```python
from build123d import *

# Parameters (mm, degrees)
SKETCH1_W           = 50
SKETCH1_H           = 10
BOSS_EXTRUDE1_DEPTH = 4
CUT_EXTRUDE1_DEPTH  = 2
CUT_EXTRUDE2_REACH  = 27.573
SKETCH3_R           = 1
CUT_EXTRUDE3_REACH  = 27.807
SKETCH4_W           = 8.712551382
SKETCH4_H           = 15.185608923
SKETCH5_W           = 19.235166375
SKETCH5_H           = 10
BOSS_EXTRUDE2_DEPTH = 4
FILLET1_R           = 10
FILLET2_R           = 2
FILLET3_R           = 2
FILLET4_R           = 2


with BuildPart() as part:
    # Sketch1 → Boss-Extrude1 (new body)
    with BuildSketch(Plane.XY):
        Rectangle(SKETCH1_W, SKETCH1_H)
    extrude(amount=BOSS_EXTRUDE1_DEPTH)

    # Sketch2 → Cut-Extrude1 (cut)
    with BuildSketch(Plane.XY.offset(4)):
        with BuildLine():
            Line((-2.254530133, 2.677142857), (-14.2, 2))
            ThreePointArc((-14.2, 2), (-16.2, 0), (-14.2, -2))
            Line((-14.2, -2), (-2.254530133, -2.677142857))
            ThreePointArc((-2.254530133, -2.677142857), (0, -3.5), (2.254530133, -2.677142857))
            Line((2.254530133, -2.677142857), (14.2, -2))
            ThreePointArc((14.2, -2), (16.2, 0), (14.2, 2))
            Line((14.2, 2), (2.254530133, 2.677142857))
            ThreePointArc((2.254530133, 2.677142857), (0, 3.5), (-2.254530133, 2.677142857))
        make_face()
    extrude(amount=-CUT_EXTRUDE1_DEPTH, mode=Mode.SUBTRACT)

    # Sketch3 → Cut-Extrude2 (cut, up to next)
    with BuildSketch(Plane.XY.offset(2), mode=Mode.PRIVATE) as cut_extrude2_sk1:
        with Locations((-14.45, 0)):
            Circle(SKETCH3_R)
    cut_extrude2_tool1 = extrude(cut_extrude2_sk1.sketch, amount=-CUT_EXTRUDE2_REACH, mode=Mode.PRIVATE) & part.part
    # Sketch3 → Cut-Extrude2 (cut, up to next)
    with BuildSketch(Plane.XY.offset(2), mode=Mode.PRIVATE) as cut_extrude2_sk2:
        with Locations(Location((14.45, 0, 0), (0, 0, 180))):
            Circle(SKETCH3_R)
    cut_extrude2_tool2 = extrude(cut_extrude2_sk2.sketch, amount=-CUT_EXTRUDE2_REACH, mode=Mode.PRIVATE) & part.part
    add(cut_extrude2_tool1.solids().sort_by_distance((-14.45, 0, 2))[0], mode=Mode.SUBTRACT)
    add(cut_extrude2_tool2.solids().sort_by_distance((14.45, 0, 2))[0], mode=Mode.SUBTRACT)

    # Sketch4 → Cut-Extrude3 (cut, up to next)
    with BuildSketch(Plane.XY.offset(4), mode=Mode.PRIVATE) as cut_extrude3_sk1:
        with Locations((-21.977833235, -0.132061848)):
            Rectangle(SKETCH4_W, SKETCH4_H)
    cut_extrude3_tool1 = extrude(cut_extrude3_sk1.sketch, amount=-CUT_EXTRUDE3_REACH, mode=Mode.PRIVATE) & part.part
    add(cut_extrude3_tool1.solids().sort_by_distance((-21.977833, -0.132062, 4))[0], mode=Mode.SUBTRACT)

    # Sketch5 → Boss-Extrude2 (add)
    with BuildSketch(Plane.XY.offset(4)):
        with Locations((34.617583188, 0)):
            Rectangle(SKETCH5_W, SKETCH5_H)
    extrude(amount=-BOSS_EXTRUDE2_DEPTH)

    # Fillet1
    fillet1_edges = [part.edges().sort_by_distance(p)[0] for p in [
        (44.235166375, 5, 2),
    ]]
    fillet(fillet1_edges, radius=FILLET1_R - 0.0001)  # a hair under: the kernel refuses the full size

    # Fillet2
    fillet2_edges = [part.edges().sort_by_distance(p)[0] for p in [
        (44.235166375, -5, 2),
    ]]
    fillet(fillet2_edges, radius=FILLET2_R)

    # Fillet3
    fillet3_edges = [part.edges().sort_by_distance(p)[0] for p in [
        (-17.621557544, 5, 2),
    ]]
    fillet(fillet3_edges, radius=FILLET3_R)

    # Fillet4
    fillet4_edges = [part.edges().sort_by_distance(p)[0] for p in [
        (-17.621557544, -5, 2),
    ]]
    fillet(fillet4_edges, radius=FILLET4_R)


solid = part.part
```
Read the model definition and answer for the solid it produces. Units are mm, in the model's axes. A direction names the side the tool comes from. Give positions to 0.01 mm unless a question says otherwise; leave off trailing zeros. Order: outer loops, then holes, each group sorted by start corner. A loop starts at its lowest first (then second) coordinate and runs counter-clockwise, first axis right, second up.
(1) Find section A-A (x = -11). Give the vertices of the cut face in (y, z), plus the area to 3 significant figures.
(2) Straight lines are drawn through the part: L1, parallel to Y at x = -14.45, z = 1.55; L2, parallel to X at y = -0.25, z = 1.9; L3, parallel to Z at x = 8, y = 2. For each, find the intervals that lie inside material, in ascending order.
(3) For faces 1 (the flat face through (0, 0, 2)), 2 (the cylindrical face through (-13.496, 0.3, 1.014)), determine the directions among +Z, -Z, +X, -X, +Y, -Y from which every point of the face is accessible in a straight line to the end or side of a thin tool.
(4) For a pull along Y with two mould halves and no side action, classify faces 3 (the flat face through (-17.622, 0, 2)), 4 (the cylindrical face through (-17.02, 4.43, 2.03)), 5 (the cylindrical face through (0, -3.5, 3)), 6 (the flat face through (-8.311, -2.334, 3.014)) as released by +Y, released by -Y, zero draft, split by the parting line, or undercut.
(5) Find section B-B (x = 4.5). Give the vertices of the cut face in (y, z).
(6) Given pin 1 (1.5 mm diameter, centred on y = 4, z = 2, fed in from +X); pin 2 (3.5 mm diameter, centred on x = -3, y = 0.5, fed in from +Z); pin 3 (3 mm diameter, centred on x = 9.5, y = -2, fed in from -Z), each flat-ended and moving along its own axis, determine where each tip first touches the part or whether it passes through.
Result sheet:
1. outline: (-5, 0) - (5, 0) - (5, 4) - (2.18, 4) - (2.18, 2) - (-2.18, 2) - (-2.18, 4) - (-5, 4) - close
1. area: 31.3 mm2
2. L1: y = -5 to -1, 1 to 5
2. L2: x = -17.62 to -15.42, -13.48 to 13.48, 15.42 to 43.04
2. L3: z = 0 to 2
3. face 1: +Z
3. face 2: +Z, -Z
4. face 3: zero draft
4. face 4: released by +Y
4. face 5: undercut
4. face 6: undercut
5. outline: (-5, 0) - (5, 0) - (5, 4) - (2.55, 4) - (2.55, 2) - (-2.55, 2) - (-2.55, 4) - (-5, 4) - close
6. pin 1: stops at x = 39.89
6. pin 2: stops at z = 2
6. pin 3: stops at z = 0
